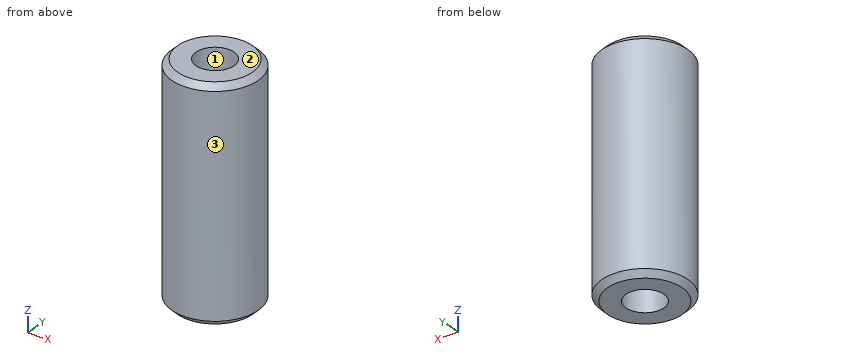
```python
from build123d import *

# Parameters (mm, degrees)
F0_R     = 9.521529
F1_DEPTH = 50.038
F2_R     = 4.212997
F3_DEPTH = 76.2
F4_SIZE  = 1.27


with BuildPart() as f1:
    # F0 (on Top) → F1 (new body)
    with BuildSketch(Plane.XY):
        with Locations((-11.465707, 22.031024)):
            Circle(F0_R)
    extrude(amount=F1_DEPTH)

    # F2 (on face) → F3 (cut)
    with BuildSketch(Plane.XY.offset(50.038)):
        with Locations((-11.465707, 22.031024)):
            Circle(F2_R)
    extrude(amount=-F3_DEPTH, mode=Mode.SUBTRACT)

    # F4
    f4_edges = [f1.edges().sort_by_distance(p)[0] for p in [
        (-20.987236, 22.031024, 0),
        (-20.987236, 22.031024, 50.038),
    ]]
    chamfer(f4_edges, length=F4_SIZE)


solid = f1.part
```
Could you check a few things on this model? Use its own coordinates, in mm. Face numbers are marked on the shaded views. Round coordinates to 2 decimals unless told otherwise and drop trailing zeros. Loops run counter-clockwise (first coordinate to the right, second up) from the corner with the lowest first, then second, coordinate; pieces in that order, holes last. Notation, with made-up numbers: M -7.75,35.25 L 7.25,35.25 A28 ccw 7.25,59.25 Z; hole C -20,73 d8. An arc over 180 degrees is marked long. Put each result on its own line as item: value.
Q1. I need wall thicknesses on probe 1 along X at (y, z) = (22.25, 26); probe 2 along Y at (x, z) = (-8.5, 32); probe 3 along Y at (x, z) = (-14.5, 28). Which ranges of each line are inside material? Lowest first, please.
Check result:
probe 1: -20.98 to -15.67, -7.26 to -1.95
probe 2: 12.98 to 19.04, 25.02 to 31.08
probe 3: 13.01 to 19.11, 24.95 to 31.06
Q2. Thinking about a two-plate mould opening in X: for the marked faces 1, 2 and 3, which applies, released by +X, released by -X, zero draft, split by the parting line, or undercut?
Check result:
face 1: undercut
face 2: zero draft
face 3: split by the parting line
Q3. Imagine slicing it at A-A (z = 29). Write out the boundary of the cut face in (x, y).
Check result:
outline: C -11.47,22.03 d19.04; hole C -11.47,22.03 d8.43
Q4. For pin 1 (6 mm diameter, centred on x = -17.5, z = 43.5, fed in from -Y); pin 2 (2 mm diameter, centred on x = -13.5, z = 15, fed in from -Y); pin 3 (1 mm diameter, centred on x = -10.5, z = 6.5, fed in from +Y), each with a flat end and sliding along its axis, tell me the tip position at first contact or that it passes through.
Check result:
pin 1: y = 13.01
pin 2: y = 12.57
pin 3: y = 31.54
